from build123d import *

# Parameters (mm, degrees)
SKETCH10_R         = 2.5
CUT_EXTRUDE1_DEPTH = 11
SKETCH11_R         = 4.5
CUT_EXTRUDE2_DEPTH = 5


with BuildPart() as part:
    # Sketch1 → Revolve1 (revolve)
    with BuildSketch(Plane.XY):
        Polygon((0, 0), (0, 10), (17.5, 10), (17.5, 7), (7, 0), align=None)
    revolve(axis=Axis((0, 0, 0), (0, 1, 0)))

    # Sketch10 → Cut-Extrude1 (cut, through all)
    with BuildSketch(Plane.XZ):
        Circle(SKETCH10_R)
    extrude(amount=-CUT_EXTRUDE1_DEPTH, mode=Mode.SUBTRACT)

    # Sketch11 → Cut-Extrude2 (cut)
    with BuildSketch(Plane.XZ):
        Circle(SKETCH11_R)
    extrude(amount=-CUT_EXTRUDE2_DEPTH, mode=Mode.SUBTRACT)


solid = part.part
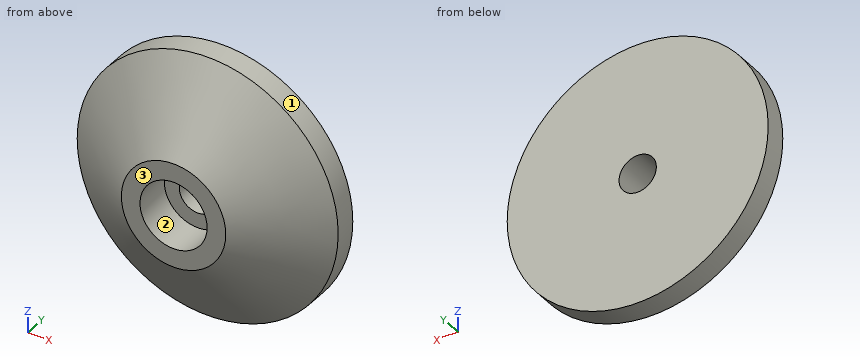
Geometry: final body of the model. Coordinates: model frame, mm. Face numbers are marked on the shaded views. Round coordinates to 2 decimals unless told otherwise and drop trailing zeros. Order: outer loops, then holes, each group sorted by start corner. A loop starts at its lowest first (then second) coordinate and runs counter-clockwise, first axis right, second up.
Q1. Pin query (flat end, axial travel): pin 1 (4 mm diameter, centred on x = 5.5, z = -10.5, fed in from -Y); pin 2 (10 mm diameter, centred on x = -0.5, z = -0.5, fed in from -Y); pin 3 (4 mm diameter, centred on x = 14, z = -2, fed in from -Y); pin 4 (2 mm diameter, centred on y = 2, z = -8.5, fed in from +X). Return the tip coordinate at first contact, or that it passes through.
Result sheet:
pin 1: stops at y = 1.9
pin 2: stops at y = 0
pin 3: stops at y = 3.43
pin 4: stops at x = 7.99
Q2. Mould query, pull axis Z, two halves, no side actions, for the marked faces 1, 2 and 3. Classes: released by +Z, released by -Z, zero draft, split by the parting line, or undercut.
Result sheet:
face 1: split by the parting line
face 2: undercut
face 3: zero draft
Q3. Material intervals for probe 1 along Z at (x, y) = (0, 7.9); probe 2 along Z at (x, y) = (1.5, 0.5); probe 3 along X at (y, z) = (6.5, -0.5), sorted ascending.
Result sheet:
probe 1: z = -17.5 to -2.5, 2.5 to 17.5
probe 2: z = -7.6 to -4.24, 4.24 to 7.6
probe 3: x = -16.74 to -2.45, 2.45 to 16.74
Q4. Section B-B, the plane x = 0. Output: boundary loops of the cut face in (y, z), and give its area (4 significant figures).
Result sheet:
outline: (0, -7) - (7, -17.5) - (10, -17.5) - (10, -2.5) - (5, -2.5) - (5, -4.5) - (0, -4.5) - close; (0, 4.5) - (5, 4.5) - (5, 2.5) - (10, 2.5) - (10, 17.5) - (7, 17.5) - (0, 7) - close
area: 206.5 mm2
Q5. Section A-A, the plane z = 0. Output: boundary loops of the cut face in (x, y).
Result sheet:
outline: (-17.5, 7) - (-7, 0) - (-4.5, 0) - (-4.5, 5) - (-2.5, 5) - (-2.5, 10) - (-17.5, 10) - close; (2.5, 5) - (4.5, 5) - (4.5, 0) - (7, 0) - (17.5, 7) - (17.5, 10) - (2.5, 10) - close
Q6. Section C-C, the plane y = 9.25. Output: boundary loops of the cut face in (x, z).
Result sheet:
outline: circle Ø35 at (0, 0); hole circle Ø5 at (0, 0)
Q7. Section D-D, the plane y = 1.5. Output: boundary loops of the cut face in (x, z).
Result sheet:
outline: circle Ø18.5 at (0, 0); hole circle Ø9 at (0, 0)
